Geometry: final body of the model. Coordinates: model frame, mm. Face numbers are marked on the shaded views. Give positions to 0.01 mm unless a question says otherwise; leave off trailing zeros. Order: outer loops, then holes, each group sorted by start corner. A loop starts at its lowest first (then second) coordinate and runs counter-clockwise, first axis right, second up. Notation, with made-up numbers: (10.5, 39) -> (69.5, 39) arc R35 ccw to (69.5, 73) -> close; hole circle Ø4 at (-19.75, -26). An arc over 180 degrees is marked (long way). One line per question, with ' | ' between items.
from build123d import *

# Parameters (mm, degrees)
F0_W     = 203.2
F0_H     = 228.6
F1_DEPTH = 76.2
F3_DEPTH = 203.2
F5_DEPTH = 171.45
F6_R     = 5.08
F7_DEPTH = 7.62


with BuildPart() as f1:
    # F0 (on Top) → F1 (new body)
    with BuildSketch(Plane.XY):
        with Locations((26.3025880603, 37.1842714906)):
            Rectangle(F0_W, F0_H)
    extrude(amount=F1_DEPTH)

    # F2 (on face) → F3 (cut)
    with BuildSketch(Plane(origin=(0, 151.4842714906, 0), x_dir=(-1, 0, 0), z_dir=(0, 1, 0))):
        Polygon((-127.9025880603, 0), (75.2974119397, 0), (-127.9025880603, 76.2), align=None)
    extrude(amount=-F3_DEPTH, mode=Mode.SUBTRACT)

    # F4 (on face) → F5 (cut)
    with BuildSketch(Plane(origin=(0, 151.4842714906, 0), x_dir=(-1, 0, 0), z_dir=(0, 1, 0))):
        with BuildLine():
            Line((-96.1709320552, 64.3006289981), (-70.0098948339, 54.4902400401))
            ThreePointArc((-70.0098948339, 54.4902400401), (-79.1150585712, 69.996380848), (-96.1709320552, 64.3006289981))
        make_face()
    extrude(amount=-F5_DEPTH, mode=Mode.SUBTRACT)

    # F6 (on face) → F7 (join)
    with BuildSketch(Plane(origin=(-9.2832425679, 0, 24.7553135144), x_dir=(0.9363291776, 0, 0.3511234416), z_dir=(0.3511234416, 0, -0.9363291776))):
        with Locations((131.4422286823, -15.679504171)):
            Circle(F6_R)
        with Locations((132.6000029427, 9.4702642467)):
            Circle(F6_R)
    extrude(amount=F7_DEPTH)


solid = f1.part
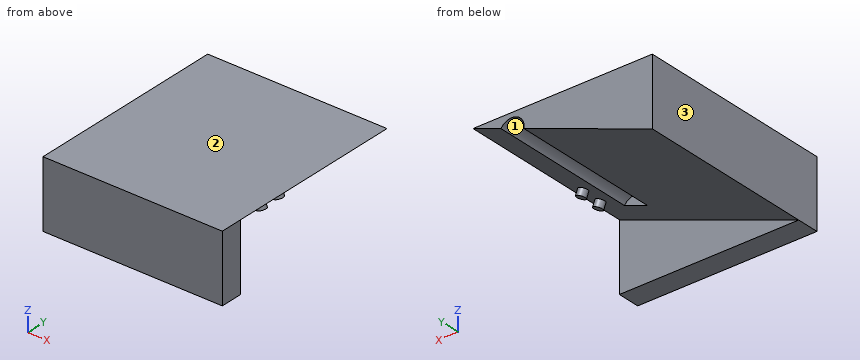
1) Section C-C on z = 35. Return loops of the section in (x, y).
Check result:
outline: (-75.3, -77.12) -> (127.9, -77.12) -> (127.9, -51.72) -> (18.04, -51.72) -> (18.04, 151.48) -> (-75.3, 151.48) -> close
2) Section A-A on x = 93. Return loops of the section in (y, z), plus the area to 3 significant figures.
Check result:
outline: (-77.12, 0) -> (-51.72, 0) -> (-51.72, 63.11) -> (-19.97, 63.11) -> (-19.97, 67.82) -> (151.48, 67.82) -> (151.48, 76.2) -> (-77.12, 76.2) -> close | area: 3,790 mm^2
3) Material intervals for probe 1 along Y at (x, z) = (92.5, 30.5); probe 2 along Z at (x, y) = (98, 137); probe 3 along Z at (x, y) = (47.5, 21), sorted ascending. Write a range as from..to.
Check result:
probe 1: y = -77.12..-51.72 | probe 2: z = 64.99..76.2 | probe 3: z = 46.05..76.2
4) Section B-B on y = 23.5. Return loops of the section in (x, z).
Check result:
outline: (-75.3, 0) -> (70.01, 54.49) arc R14.28 cw to (96.17, 64.3) -> (127.9, 76.2) -> (-75.3, 76.2) -> close
5) Section D-D on z = 50.5. Return loops of the section in (x, y), plus the area to 3 significant figures.
Check result:
outline: (-75.3, -77.12) -> (127.9, -77.12) -> (127.9, -51.72) -> (59.37, -51.72) -> (59.37, 151.48) -> (-75.3, 151.48) -> close | area: 32,500 mm^2
6) Pull-direction query (X, two-part tool) for the marked faces 1, 2 and 3; classes: +X half, -X half, draft (parallel to the pull), parting line (faces both ways), or undercut.
Check result:
face 1: undercut | face 2: draft | face 3: -X half
7) Contact query for flat-ended pins moving along their axis: pin 1 Ø1 at (x, y) = (-11, 2.5) entering from -Z; pin 2 Ø13 at (x, z) = (78.5, 59) entering from +Y; pin 3 Ø3 at (x, y) = (-12.5, 99.5) entering from -Z. Output: stop coordinate, or through.
Check result:
pin 1: stops at z = 23.92 | pin 2: stops at y = -19.97 | pin 3: stops at z = 22.99
